Model file for the job. Use its own axes, mm. Face numbers are marked on the shaded views. A direction names the side the tool comes from. Round coordinates to 2 decimals unless told otherwise and drop trailing zeros. Loops run counter-clockwise (first coordinate to the right, second up) from the corner with the lowest first, then second, coordinate; pieces in that order, holes last. Notation, with made-up numbers: M 79.5,69.25 L 88.5,69.25 A22 cw 88.5,90.25 Z; hole C -25.75,61 d5. An arc over 180 degrees is marked long. Answer in a Markdown table with one row per item.
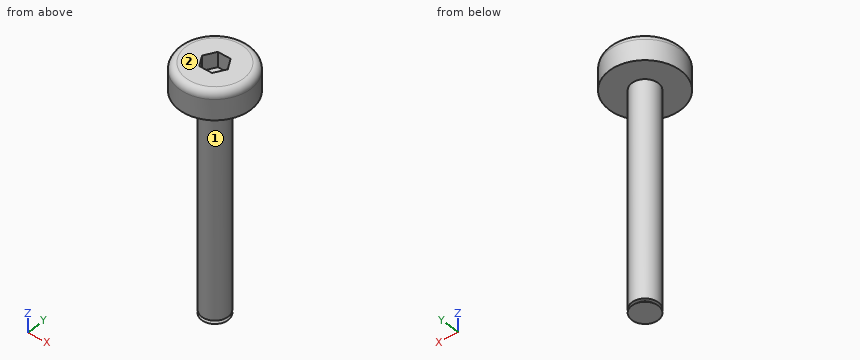
from build123d import *

# Parameters (mm, degrees)
F_0090_CYLINDER_SKETCH_R    = 3.25
F_0090_CYLINDER_DEPTH       = 2.5
F_0091_FILLET_R             = 0.625
F_0092_EXTRUDE_DEPTH        = 1.385
F_0092_EXTRUDE_ROTATE_ANGLE = 120
F_0095_CYLINDER_SKETCH_R    = 1.2
F_0095_CYLINDER_DEPTH       = 19.7
F_0096_CONE_ROTATE_ANGLE    = 90


with BuildPart() as part:
    # 0090_cylinder_Sketch → 0090_cylinder (new body)
    with BuildSketch(Plane.XY):
        Circle(F_0090_CYLINDER_SKETCH_R)
    extrude(amount=F_0090_CYLINDER_DEPTH)

    # 0091_fillet
    f_0091_fillet_edges = [part.edges().sort_by_distance(p)[0] for p in [
        (-3.25, 0, 2.5),
    ]]
    fillet(f_0091_fillet_edges, radius=F_0091_FILLET_R)


with BuildPart() as body_2:
    # 0092_extrude_Sketch → 0092_extrude (new body)
    with BuildSketch(Plane.XY):
        Polygon((0, 0), (1.154700538, 0), (1.732050808, 1), (1.154700538, 2), (0, 2), (-0.577350269, 1), align=None)
    extrude(amount=F_0092_EXTRUDE_DEPTH)


with BuildPart() as body_2_1:
    # 0092_extrude_Rotate: read off the stored shape, not the designer's step
    # 0092_extrude_Rotate: moved
    add(body_2.part.rotate(Axis((0, 0, 0), (0, 0, 1)), F_0092_EXTRUDE_ROTATE_ANGLE))


with BuildPart() as body_2_2:
    # 0092_extrude_Translate: moved
    add(body_2_1.part.moved(Location((1.154700538, 0, 1.125))))


with BuildPart() as part_1:
    add(part.part)

    # 0094_sub: cut body 2
    add(body_2_2.part, mode=Mode.SUBTRACT)


with BuildPart() as body_2_2_1:
    # 0095_cylinder_Sketch → 0095_cylinder (new body)
    with BuildSketch(Plane.XY):
        Circle(F_0095_CYLINDER_SKETCH_R)
    extrude(amount=F_0095_CYLINDER_DEPTH)


with BuildPart() as body_2_2_2:
    # 0095_cylinder_Translate: moved
    add(body_2_2_1.part.moved(Location((0, 0, -19.7))))


with BuildPart() as body_3:
    # 0096_cone_Sketch → 0096_cone (revolve)
    with BuildSketch(Plane.XY, mode=Mode.PRIVATE) as f_0096_cone_sk:
        Polygon((0, 0), (1.2, 0), (0.9, 0.3), (0, 0.3), align=None)
    revolve(f_0096_cone_sk.sketch.rotate(Axis((0, -100, 0), (0, 1, 0)), 90), axis=Axis((0, -100, 0), (0, 1, 0)))


with BuildPart() as body_3_1:
    # 0096_cone_Rotate: moved
    add(body_3.part.rotate(Axis((0, 0, 0), (1, 0, 0)), F_0096_CONE_ROTATE_ANGLE))


with BuildPart() as body_3_2:
    # 0096_cone_Translate: moved
    add(body_3_1.part.moved(Location((0, 0, -20))))


with BuildPart() as body_2_2_3:
    add(body_2_2_2.part)

    # 0098_add: union body 3
    add(body_3_2.part)


with BuildPart() as part_2:
    add(part_1.part)

    # 0099_add: union body 2 2
    add(body_2_2_3.part)


solid = part_2.part
1. Saw through at A-A (x = 0). Write the cut outline in (y, z) (3 decimals), and give its area (3 significant figures).
Verdict:
| item | result |
|---|---|
| outline | M -3.25,0 L -1.2,0 L -1.2,-19.7 L -0.9,-19.7 L -1.2,-20 L 1.2,-20 L 0.9,-19.7 L 1.2,-19.7 L 1.2,0 L 3.25,0 L 3.25,1.875 A0.625 ccw 2.625,2.5 L 1,2.5 L 1,1.125 L -1,1.125 L -1,2.5 L -2.625,2.5 A0.625 ccw -3.25,1.875 Z |
| area | 61.2 mm² |
2. Saw through at B-B (z = 0.5). Write the cut outline in (x, y), and give its area (3 significant figures).
Verdict:
| item | result |
|---|---|
| outline | C 0,0 d6.5 |
| area | 33.2 mm² |
3. Wall check: probe 1 along Y at (x, z) = (0, -17.25); probe 2 along Z at (x, y) = (0.5, -1.5); probe 3 along X at (y, z) = (-0.5, -1.25). Give the ranges that are in metal, low to high.
Verdict:
| item | result |
|---|---|
| probe 1 | y = -1.2 to 1.2 |
| probe 2 | z = 0 to 2.5 |
| probe 3 | x = -1.09 to 1.09 |
4. Saw through at C-C (z = -9.75). Write the cut outline in (x, y), and give its area (3 significant figures).
Verdict:
| item | result |
|---|---|
| outline | C 0,0 d2.4 |
| area | 4.52 mm² |
5. Pin check, flat tips, straight feed: pin 1 (1 mm diameter, centred on x = 0.5, z = -1, fed in from -Y); pin 2 (1 mm diameter, centred on x = 0.5, y = 0, fed in from +Z) (3 decimals); pin 3 (1.5 mm diameter, centred on x = -2.5, z = -1.5, fed in from -Y). Stop position of each tip, or through.
Verdict:
| item | result |
|---|---|
| pin 1 | stops at y = -1.2 |
| pin 2 | stops at z = 1.125 |
| pin 3 | passes through |
6. Tool access for the marked faces 1 and 2: list every direction of +Z, -Z, +X, -X, +Y, -Y with a clear straight run to the whole face (end or side of a thin tool).
Verdict:
| item | result |
|---|---|
| face 1 | -Z |
| face 2 | +Z, +X, -X, +Y, -Y |
